Build history of the part. All positions in model axes, mm. A direction names the side the tool comes from. Round coordinates to 2 decimals unless told otherwise and drop trailing zeros. Loops run counter-clockwise (first coordinate to the right, second up) from the corner with the lowest first, then second, coordinate; pieces in that order, holes last. Notation, with made-up numbers: (11.25, 17.5) - (61.25, 17.5) arc R10 ccw to (61.25, 26.5) - close; hole circle Ø5 at (30.25, 79). An arc over 180 degrees is marked (long way). Put each result on its own line as item: value. Start each with the question number.
from build123d import *

# Parameters (mm, degrees)
BOSS_EXTRUDE1_DEPTH = 11.5
SKETCH4_W           = 12.8
SKETCH4_H           = 11
BOSS_EXTRUDE2_DEPTH = 11
BOSS_EXTRUDE2_TAPER = 5
SKETCH5_R           = 4.5
SKETCH5_R_2         = 3.5
BOSS_EXTRUDE3_DEPTH = 11


with BuildPart() as part:
    # Sketch2 → Boss-Extrude1 (new body)
    with BuildSketch(Plane(origin=(0, 0, 0), x_dir=(1, 0, 0), z_dir=(0, 1, 0))):
        Polygon((-6, -5), (-6, -7.5), (6, -7.5), (6, 7.5), (-6, 7.5), (-6, 5), (-5, 5), (-5, -5), align=None)
    extrude(amount=BOSS_EXTRUDE1_DEPTH)

    # Sketch4 → Boss-Extrude2 (add)
    with BuildSketch(Plane(origin=(6, 0, 0), x_dir=(0, 0, -1), z_dir=(1, 0, 0))):
        with Locations((0, 5.75)):
            Rectangle(SKETCH4_W, SKETCH4_H)
    extrude(amount=BOSS_EXTRUDE2_DEPTH, taper=BOSS_EXTRUDE2_TAPER)

    # Sketch5 → Boss-Extrude3 (add)
    with BuildSketch(Plane(origin=(17, 0, 0), x_dir=(0, 0, -1), z_dir=(1, 0, 0))):
        with Locations((0, 5.75)):
            Circle(SKETCH5_R)
        with Locations((0, 5.75)):
            Circle(SKETCH5_R_2, mode=Mode.SUBTRACT)
    extrude(amount=BOSS_EXTRUDE3_DEPTH)


solid = part.part
Item 1: Drill centre lines: probe 1 along Y at (x, z) = (25.5, 0); probe 2 along X at (y, z) = (7, 4.75); probe 3 along Z at (x, y) = (23.5, 6). Where is each one in solid material? Low to high. Write a range as [from, to].
Item 2: Drop flat-ended pins along their axis: pin 1 Ø1 at (x, z) = (14, 4) entering from +Y; pin 2 Ø3 at (x, z) = (8.5, -2.5) entering from +Y; pin 3 Ø3.5 at (y, z) = (4.5, -1) entering from +X. Give the stop position or say it passes through.
Item 3: Which spindle directions (+Z, -Z, +X, -X, +Y, -Y) get a long thin tool onto all of the face, cutting with end or side? Do faces 5 (the cylindrical face through (22.423, 2.333, 0.759)), 6 (the flat face through (0, 6, -7.5)), 7 (the flat face through (-5.5, 5.7, -5)). Say none if no direction does.
Item 4: Slice it at A-A (x = 21). Give the cut face in (y, z), plus the area to 3 significant figures.
Item 5: Two-plate mould, pull along Z, no slides. Class faces 1 (the flat face through (17, 6, 0)), 2 (the cylindrical face through (22.42, 1.36, 0.98)), 3 (the flat face through (-5.5, 5.7, 5)), 4 (the flat face through (-6, 6, -6)): pulls with the +Z half, pulls with the -Z half, needs draft (parallel to the pull), parting line crosses it, or undercut.
Computed values:
1. probe 1: y = [1.25, 2.25], [9.25, 10.25]
1. probe 2: x = [-5, 17]
1. probe 3: z = [-4.49, -3.49], [3.49, 4.49]
2. pin 1: stops at y = 10.59
2. pin 2: stops at y = 11.16
2. pin 3: stops at x = 17
3. face 5: +X
3. face 6: -Z, +X, -X, +Y, -Y
3. face 7: -X, +Y, -Y
4. outline: circle Ø9 at (5.75, 0); hole circle Ø7 at (5.75, 0)
4. area: 25.1 mm^2
5. face 1: undercut
5. face 2: parting line crosses it
5. face 3: undercut
5. face 4: needs draft
